```python
from build123d import *

# Parameters (mm, degrees)
F1_DEPTH  = 20
F2_DEPTH  = 20
F4_DEPTH  = 15
F5_W      = 44
F5_H      = 59
F5_W_2    = 34
F5_H_2    = 49
F7_DEPTH  = 25
F8_DEPTH  = 20
F6_W      = 48
F6_H      = 9
F9_DEPTH  = 45
F10_W     = 1.5
F10_H     = 49
F11_DEPTH = 18
F12_W     = 49
F12_H     = 20
F13_DEPTH = 4
F14_W     = 49
F14_H     = 1
F15_DEPTH = 39
F16_R     = 2.25
F16_R_2   = 1.25
F17_DEPTH = 10
F18_W     = 5.25
F18_H     = 5.25
F19_DEPTH = 15


with BuildPart() as f1:
    # F0 (on Top) → F1 (new body)
    with BuildSketch(Plane.XY):
        Polygon((0, 66), (0, 9), (9, 0), (51, 0), (60, 9), (60, 66), (51, 75), (9, 75), align=None)
    extrude(amount=F1_DEPTH)

    # F0 (on Top) → F2 (join)
    with BuildSketch(Plane.XY):
        Polygon((0, 66), (0, 9), (9, 0), (51, 0), (60, 9), (60, 66), (51, 75), (9, 75), align=None)
    extrude(amount=F2_DEPTH)

    # F3 (on face) → F4 (cut)
    with BuildSketch(Plane.XY.offset(20)):
        Polygon((5.2071067812, 71.2071067812), (3.7928932188, 69.7928932188), (5.2071067812, 68.3786796564), (6.6213203436, 69.7928932188), align=None)
        Polygon((6.6213203436, 69.7928932188), (5.2071067812, 68.3786796564), (2.3786796564, 65.5502525317), (3.4393398282, 64.4895923599), (10.5104076401, 71.5606601718), (9.4497474683, 72.6213203436), align=None)
        Polygon((2.3786796564, 9.4497474683), (5.2071067812, 6.6213203436), (6.6213203436, 5.2071067812), (9.4497474683, 2.3786796564), (10.8639610307, 3.7928932188), (3.7928932188, 10.8639610307), align=None)
        Polygon((5.2071067812, 6.6213203436), (3.7928932188, 5.2071067812), (5.2071067812, 3.7928932188), (6.6213203436, 5.2071067812), align=None)
        Polygon((53.3786796564, 5.2071067812), (54.7928932188, 3.7928932188), (56.2071067812, 5.2071067812), (54.7928932188, 6.6213203436), align=None)
        Polygon((50.5502525317, 2.3786796564), (53.3786796564, 5.2071067812), (54.7928932188, 6.6213203436), (57.6213203436, 9.4497474683), (56.5606601718, 10.5104076401), (49.4895923599, 3.4393398282), align=None)
        Polygon((54.7928932188, 68.3786796564), (53.3786796564, 69.7928932188), (50.5502525317, 72.6213203436), (49.4895923599, 71.5606601718), (56.5606601718, 64.4895923599), (57.6213203436, 65.5502525317), align=None)
        Polygon((56.2071067812, 69.7928932188), (54.7928932188, 71.2071067812), (53.3786796564, 69.7928932188), (54.7928932188, 68.3786796564), align=None)
    extrude(amount=-F4_DEPTH, mode=Mode.SUBTRACT)

    # F5 (on face) → F7 (join)
    with BuildSketch(Plane.XY.offset(20)):
        with Locations((30, 37.5)):
            Rectangle(F5_W, F5_H)
        with Locations((30, 37.5)):
            Rectangle(F5_W_2, F5_H_2, mode=Mode.SUBTRACT)
        with Locations((30, 37.5)):
            Rectangle(F5_W_2, F5_H_2)
    extrude(amount=-F7_DEPTH)

    # F5 (on face) → F8 (cut)
    with BuildSketch(Plane.XY.offset(20)):
        with Locations((30, 37.5)):
            Rectangle(F5_W_2, F5_H_2)
    extrude(amount=-F8_DEPTH, mode=Mode.SUBTRACT)

    # F6 (on face) → F9 (cut)
    with BuildSketch(Plane.YZ.offset(60)):
        with Locations((37.5, 7.5)):
            Rectangle(F6_W, F6_H)
    extrude(amount=-F9_DEPTH, mode=Mode.SUBTRACT)

    # F10 (on face) → F11 (cut)
    with BuildSketch(Plane.XY.offset(20)):
        with Locations((54.25, 37.5)):
            Rectangle(F10_W, F10_H)
    extrude(amount=-F11_DEPTH, mode=Mode.SUBTRACT)

    # F12 (on face) → F13 (cut)
    with BuildSketch(Plane.YZ.offset(13)):
        with Locations((37.5, 10)):
            Rectangle(F12_W, F12_H)
    extrude(amount=-F13_DEPTH, mode=Mode.SUBTRACT)

    # F14 (on face) → F15 (join)
    with BuildSketch(Plane.YZ.offset(9)):
        with Locations((37.5, 11.5)):
            Rectangle(F14_W, F14_H)
    extrude(amount=F15_DEPTH)

    # F16 (on face) → F17 (cut)
    with BuildSketch(Plane.XY.offset(20)):
        with Locations((18, 7)):
            Circle(F16_R)
        with Locations((28, 68)):
            Circle(F16_R)
        with Locations((5, 37.5)):
            Circle(F16_R_2)
        with Locations((38, 7)):
            Circle(F16_R)
    extrude(amount=-F17_DEPTH, mode=Mode.SUBTRACT)

    # F18 (on face) → F19 (cut)
    with BuildSketch(Plane.XZ):
        with Locations((30, 12.375)):
            Rectangle(F18_W, F18_H)
    extrude(amount=-F19_DEPTH, mode=Mode.SUBTRACT)


solid = f1.part
```
Source: CAD feature listing. Evaluate the final solid. Frame: model axes, mm. A direction names the side the tool comes from. Give positions to 0.01 mm unless a question says otherwise; leave off trailing zeros. Write each loop counter-clockwise with the first axis right and the second up, starting at its lowest first coordinate (ties: lowest second). Pieces come first, ordered by that corner, then holes.
1. First-contact query: pin 1 (5.5 mm diameter, centred on x = 34, z = -3, fed in from -Y); pin 2 (6 mm diameter, centred on y = 5.5, z = 13, fed in from +X); pin 3 (1.6 mm diameter, centred on x = 54, z = 6.5, fed in from -Y). Flat tips, straight axial feed; report the tip coordinate or a pass-through.
2. Material intervals for line 1 along Y through (x, z) = (38, 15.25); line 2 along Y through (x, z) = (28, 17.5); line 3 along Y through (x, z) = (13.5, 1), sorted ascending.
3. Section query A-A (y = 27). Return the cut outline in (x, z).
4. Section query B-B (x = 38). Return the cut outline in (y, z), then the cut area to 3 significant figures.
5. Section query C-C (y = 63). Return the cut outline in (x, z).
6. Pull-direction query (Y, two-part tool) for faces 4 (the face through (6.93, 67.98, 12.6)), 5 (the face through (30, 75, 10)), 6 (the face through (0, 38, 10)); classes: +Y half, -Y half, draft (parallel to the pull), parting line (faces both ways), or undercut.
7. Access query for faces 1 (the face through (8, 37, -2)), 2 (the face through (52.98, 68.07, 12.6)), 3 (the face through (50, 13.5, 7)). Directions: +Z, -Z, +X, -X, +Y, -Y. A direction counts if a zero-diameter tool reaches every point of the face in a straight line with its end or side. Return the directions, or none.
Output values:
1. pin 1: stops at y = 8
1. pin 2: stops at x = 59.5
1. pin 3: stops at y = 2.2
2. line 1: y = 0 to 4.75, 9.25 to 13, 62 to 75
2. line 2: y = 0 to 13, 62 to 65.75, 70.25 to 75
2. line 3: y = 0 to 13, 62 to 75
3. outline: (0, 0) - (8, 0) - (8, -5) - (52, -5) - (52, 0) - (60, 0) - (60, 3) - (55, 3) - (55, 2) - (53.5, 2) - (53.5, 3) - (47, 3) - (47, 0) - (9, 0) - (9, 11) - (48, 11) - (48, 12) - (53.5, 12) - (53.5, 20) - (47, 20) - (47, 12) - (9, 12) - (9, 20) - (0, 20) - close; (55, 12) - (60, 12) - (60, 20) - (55, 20) - close
4. outline: (0, 0) - (8, 0) - (8, -5) - (67, -5) - (67, 0) - (75, 0) - (75, 20) - (62, 20) - (62, 12) - (13, 12) - (13, 20) - (9.25, 20) - (9.25, 10) - (4.75, 10) - (4.75, 20) - (0, 20) - close; hole (13, 0) - (62, 0) - (62, 11) - (13, 11) - close
4. area: 819 mm2
5. outline: (0, 0) - (8, 0) - (8, -5) - (52, -5) - (52, 0) - (60, 0) - (60, 20) - (0, 20) - close
6. face 4: undercut
6. face 5: +Y half
6. face 6: draft
7. face 1: -Z, -X, +Y, -Y
7. face 2: +Z
7. face 3: +X
